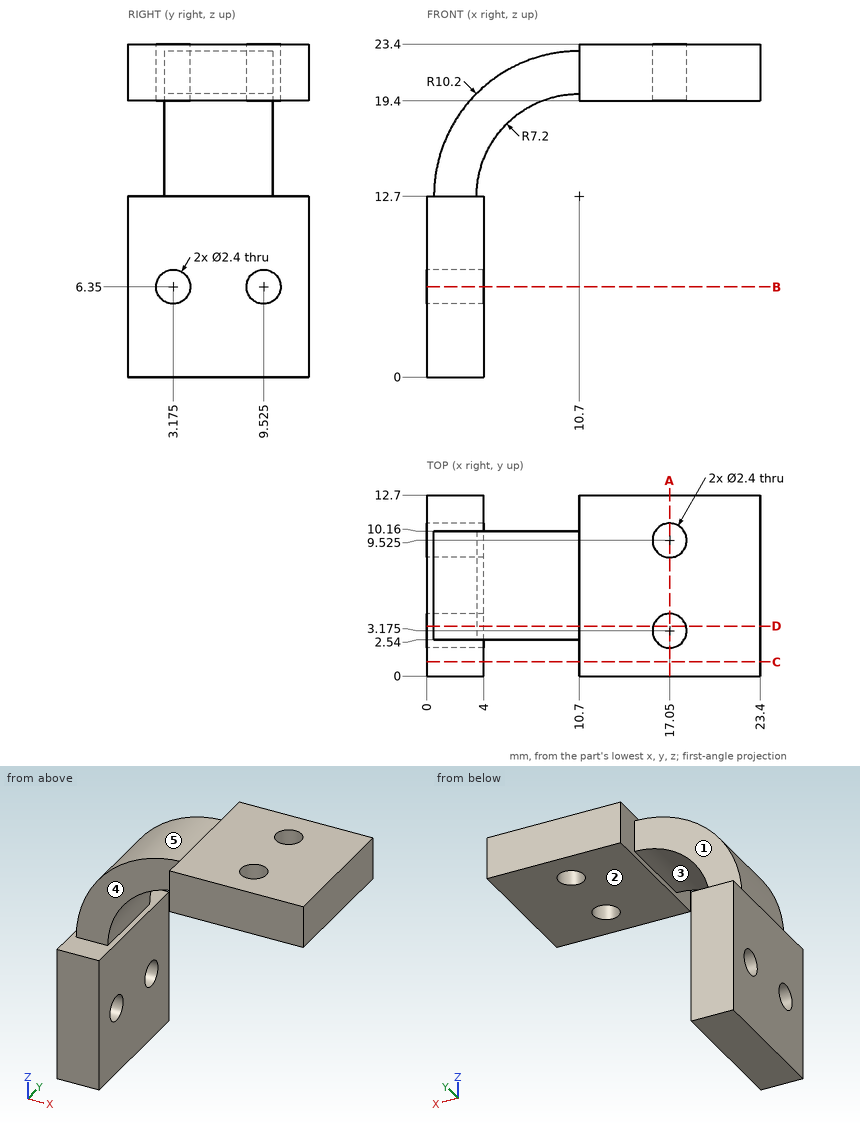
Geometry check sheet. Reference: drawing and pictorial views, mm from the part's lowest x, y, z. A direction names the side the tool comes from. Give positions to 0.01 mm unless a question says otherwise; leave off trailing zeros. Write each loop counter-clockwise with the first axis right and the second up, starting at its lowest first coordinate (ties: lowest second). Pieces come first, ordered by that corner, then holes. Notation, with made-up numbers: (14.5, 11) -> (47.5, 11) arc R26 ccw to (47.5, 35) -> close; hole circle Ø11 at (1, 36). An arc over 180 degrees is marked (long way). One line per item, written item: value. Start each with the question number.
Item 1: Tool access check on the marked faces 1, 2, 3, 4 and 5. Record the directions out of +Z, -Z, +X, -X, +Y, -Y that give a thin tool (end or side, any length) a straight path to the whole face; none if there is none.
Item 2: Section check D-D on y = 3.5. Record the cut outline in (x, z).
Item 3: Section check B-B on z = 6.35. Record the cut outline in (x, y) (3 decimals), then the cut area to 3 significant figures.
Item 4: Material ranges on probe 1 along Y at (x, z) = (1.5, 6.35) (3 decimals); probe 2 along Y at (x, z) = (10.5, 20.75); probe 3 along X at (y, z) = (2.25, 8), recorded low to high. Write a range as from..to.
Item 5: Gauge pin test, flat ends, axial feed: pin 1 (4 mm diameter, centred on y = 9.5, z = 9.5, fed in from +X); pin 2 (3 mm diameter, centred on x = 2.5, y = 9.5, fed in from +Z); pin 3 (4 mm diameter, centred on x = 15, y = 4.5, fed in from -Z). Record the tip position at first contact, or that the pin passes through.
Item 6: Section check C-C on y = 1. Record the cut outline in (x, z).
Item 7: Section check A-A on x = 17.05. Record the cut outline in (y, z) (3 decimals), then the cut area to 3 significant figures.
Results list:
1. face 1: +Z, -X, +Y
1. face 2: -Z, +X, +Y, -Y
1. face 3: +Y, -Y
1. face 4: +Z, -X, -Y
1. face 5: +Z, -X, +Y, -Y
2. outline: (0, 0) -> (4, 0) -> (4, 5.19) -> (0, 5.19) -> close; (0, 7.51) -> (4, 7.51) -> (4, 12.7) -> (3.5, 12.7) arc R7.2 cw to (10.7, 19.9) -> (10.7, 19.4) -> (15.89, 19.4) -> (15.89, 23.4) -> (10.7, 23.4) -> (10.7, 22.9) arc R10.2 ccw to (0.5, 12.7) -> (0, 12.7) -> close; (18.21, 19.4) -> (23.4, 19.4) -> (23.4, 23.4) -> (18.21, 23.4) -> close
3. outline: (0, 0) -> (4, 0) -> (4, 1.975) -> (0, 1.975) -> close; (0, 4.375) -> (4, 4.375) -> (4, 8.325) -> (0, 8.325) -> close; (0, 10.725) -> (4, 10.725) -> (4, 12.7) -> (0, 12.7) -> close
3. area: 31.6 mm²
4. probe 1: 0..1.975, 4.375..8.325, 10.725..12.7
4. probe 2: 2.54..10.16
4. probe 3: 0..4
5. pin 1: x = 4
5. pin 2: z = 20.39
5. pin 3: z = 19.4
6. outline: (0, 0) -> (4, 0) -> (4, 12.7) -> (0, 12.7) -> close; (10.7, 19.4) -> (23.4, 19.4) -> (23.4, 23.4) -> (10.7, 23.4) -> close
7. outline: (0, 19.4) -> (1.975, 19.4) -> (1.975, 23.4) -> (0, 23.4) -> close; (4.375, 19.4) -> (8.325, 19.4) -> (8.325, 23.4) -> (4.375, 23.4) -> close; (10.725, 19.4) -> (12.7, 19.4) -> (12.7, 23.4) -> (10.725, 23.4) -> close
7. area: 31.6 mm²
